Read the model definition and answer for the solid it produces. Units are mm, in the model's axes. Round coordinates to 2 decimals unless told otherwise and drop trailing zeros. Loops run counter-clockwise (first coordinate to the right, second up) from the corner with the lowest first, then second, coordinate; pieces in that order, holes last. Notation, with made-up numbers: (40.5, 48.5) -> (76.5, 48.5) arc R22 cw to (76.5, 84.5) -> close; hole circle Ø8 at (36, -31). An arc over 180 degrees is marked (long way). Put each result on its own line as item: value.
from build123d import *

# Parameters (mm, degrees)
SKETCH1_W           = 83
SKETCH1_H           = 83
BOSS_EXTRUDE1_DEPTH = 3
SKETCH2_W           = 13
SKETCH2_H           = 25
CUT_EXTRUDE1_DEPTH  = 3
CHAMFER1_SIZE       = 3.5
SKETCH3_W           = 15
SKETCH3_H           = 3
SKETCH3_W_2         = 3
SKETCH3_H_2         = 15
BOSS_EXTRUDE2_DEPTH = 3
SKETCH5_W           = 175
SKETCH5_H           = 3
BOSS_EXTRUDE4_DEPTH = 1
SKETCH6_W           = 3
SKETCH6_H           = 612
BOSS_EXTRUDE5_DEPTH = 1


with BuildPart() as part:
    # Sketch1 → Boss-Extrude1 (new body)
    with BuildSketch(Plane.XY):
        Rectangle(SKETCH1_W, SKETCH1_H)
    extrude(amount=BOSS_EXTRUDE1_DEPTH)

    # Sketch2 → Cut-Extrude1 (cut)
    with BuildSketch(Plane.XY.offset(3)):
        with Locations((0, 25.5)):
            Rectangle(SKETCH2_W, SKETCH2_H)
        with Locations((0, -25.5)):
            Rectangle(SKETCH2_W, SKETCH2_H)
    extrude(amount=-CUT_EXTRUDE1_DEPTH, mode=Mode.SUBTRACT)

    # Chamfer1
    chamfer1_edges = [part.edges().sort_by_distance(p)[0] for p in [
        (-41.5, 41.5, 1.5),
        (41.5, 41.5, 1.5),
        (41.5, -41.5, 1.5),
        (-41.5, -41.5, 1.5),
    ]]
    chamfer(chamfer1_edges, length=CHAMFER1_SIZE)

    # Sketch3 → Boss-Extrude2 (add)
    with BuildSketch(Plane.XY.offset(3)):
        with Locations((-11, -1)):
            Rectangle(SKETCH3_W, SKETCH3_H)
        with Locations((25, 22)):
            Rectangle(SKETCH3_W_2, SKETCH3_H_2)
    extrude(amount=BOSS_EXTRUDE2_DEPTH)

    # Sketch5 → Boss-Extrude4 (add)
    with BuildSketch(Plane.XZ.offset(2.5)):
        with Locations((-91, 4.5)):
            Rectangle(SKETCH5_W, SKETCH5_H)
    extrude(amount=BOSS_EXTRUDE4_DEPTH)

    # Sketch6 → Boss-Extrude5 (add)
    with BuildSketch(Plane(origin=(26.5, 0, 0), x_dir=(0, 0, -1), z_dir=(1, 0, 0))):
        with Locations((-4.5, -276.5)):
            Rectangle(SKETCH6_W, SKETCH6_H)
    extrude(amount=BOSS_EXTRUDE5_DEPTH)


solid = part.part
Item 1: The part is cut by section A-A (z = 2). Determine the outline of the cut face in (x, y), then the cut area to 3 significant figures.
Derived:
outline: (-41.5, -38) -> (-38, -41.5) -> (38, -41.5) -> (41.5, -38) -> (41.5, 38) -> (38, 41.5) -> (-38, 41.5) -> (-41.5, 38) -> close; hole (-6.5, -38) -> (6.5, -38) -> (6.5, -13) -> (-6.5, -13) -> close; hole (-6.5, 13) -> (6.5, 13) -> (6.5, 38) -> (-6.5, 38) -> close
area: 6,210 mm^2
Item 2: The part is cut by section C-C (y = -472). Determine the outline of the cut face in (x, z).
Derived:
outline: (26.5, 3) -> (27.5, 3) -> (27.5, 6) -> (26.5, 6) -> close
Item 3: Flat-ended cylindrical pins translate along their axes: pin 1 Ø1.5 at (y, z) = (-345, 5) entering from +X; pin 2 Ø1.5 at (x, z) = (24.5, 4) entering from +Y; pin 3 Ø1.5 at (x, z) = (-110, 4.5) entering from +Y. Find the tip coordinate at first contact, or state that the pin passes through.
Derived:
pin 1: stops at x = 27.5
pin 2: stops at y = 29.5
pin 3: stops at y = -2.5
Item 4: The part is cut by section B-B (x = -49). Determine the outline of the cut face in (y, z).
Derived:
outline: (-3.5, 3) -> (-2.5, 3) -> (-2.5, 6) -> (-3.5, 6) -> close
Item 5: Find the intervals of material crossed by line 1 along X through (y, z) = (6.5, 1.45); line 2 along X through (y, z) = (-213.5, 3.3); line 3 along Y through (x, z) = (-98.5, 3.4), in increasing order.
Derived:
line 1: x = -41.5 to 41.5
line 2: x = 26.5 to 27.5
line 3: y = -3.5 to -2.5
